Geometry check sheet. Reference: drawing and pictorial views, mm from the part's lowest x, y, z. A direction names the side the tool comes from. Coordinates: 2 decimals unless noted, no trailing zeros. Write each loop counter-clockwise with the first axis right and the second up, starting at its lowest first coordinate (ties: lowest second). Pieces come first, ordered by that corner, then holes. Notation, with made-up numbers: M 29.25,4.25 L 70.25,4.25 A36 ccw 70.25,39.25 Z; hole C 39,-22.75 d7. An arc over 180 degrees is marked long. One line per item, written item: value.
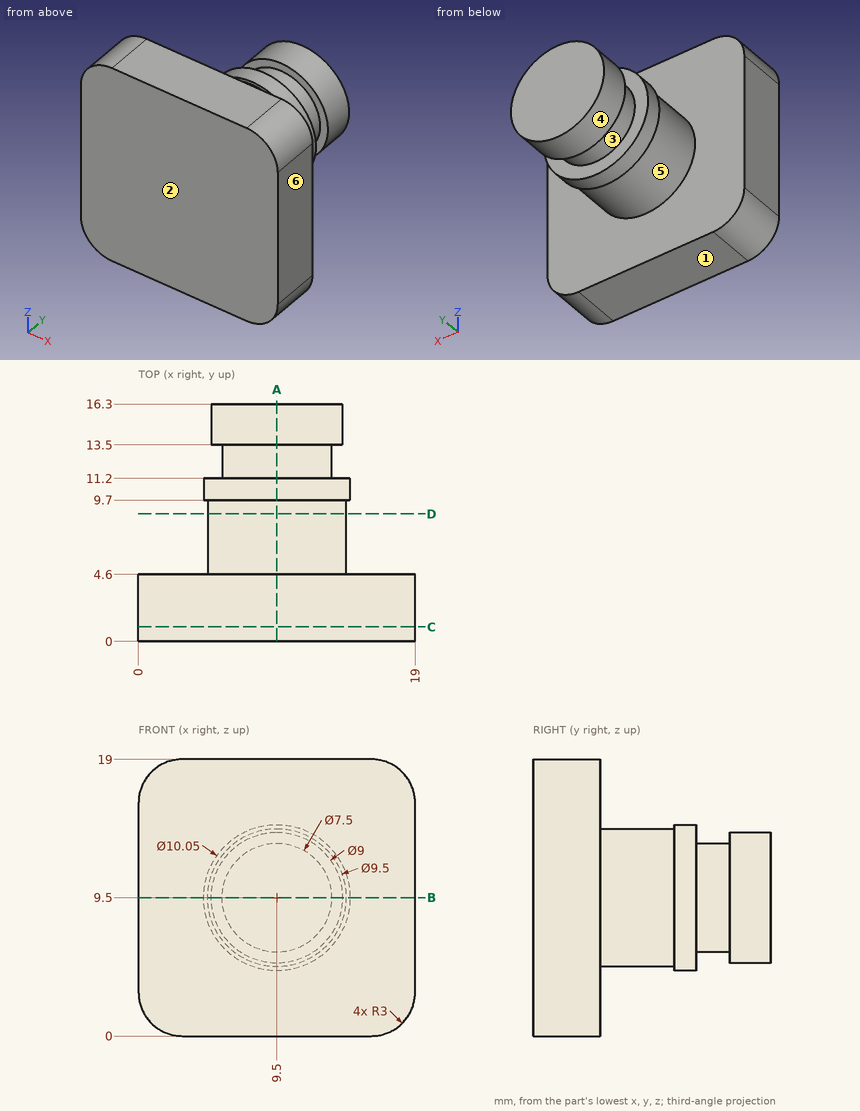
Item 1: Draft check along Y on the marked faces 1, 2 and 3. Enter one of: released by +Y, released by -Y, zero draft, split by the parting line, or undercut.
The answers:
face 1: zero draft
face 2: released by -Y
face 3: undercut
Item 2: Access from +Z, -Z, +X, -X, +Y, -Y to the whole of each face (thin tool, end or side, straight path). Record for the marked faces 4, 5 and 6.
The answers:
face 4: +Y
face 5: none
face 6: +Z, -Z, +X, +Y, -Y
Item 3: Go/stop test with flat-tipped pins: P1, Ø5, axis at x = 11, y = 2.5, coming from the -Z side; P2, Ø4, axis at x = 16.5, y = 12, coming from the -Z side; P3, Ø1, axis at x = 8.5, y = 9.5, coming from the +Z side; P4, Ø5, axis at y = 13, z = 10.5, coming from the +X side (3 decimals). Record where each tip stops, or that it passes through.
The answers:
P1: stops at z = 0
P2: passes through
P3: stops at z = 14.5
P4: stops at x = 14.525
Item 4: Cross-section at C-C, the plane y = 1. Enter the section's corners in (x, z), and give its area (3 significant figures).
The answers:
outline: M 0,3 A3 ccw 3,0 L 16,0 A3 ccw 19,3 L 19,16 A3 ccw 16,19 L 3,19 A3 ccw 0,16 Z
area: 353 mm²
Item 5: Cross-section at B-B, the plane z = 9.5. Enter the section's corners in (x, y) (3 decimals).
The answers:
outline: M 0,0 L 19,0 L 19,4.6 L 14.25,4.6 L 14.25,9.7 L 14.525,9.7 L 14.525,11.2 L 13.25,11.2 L 13.25,13.5 L 14,13.5 L 14,16.3 L 5,16.3 L 5,13.5 L 5.75,13.5 L 5.75,11.2 L 4.475,11.2 L 4.475,9.7 L 4.75,9.7 L 4.75,4.6 L 0,4.6 Z
Item 6: Scan lines: line 1 (Y direction, x = 5.5, z = 16.5); line 2 (X direction, y = 5, z = 11.5); line 3 (Z direction, x = 9.25, y = 10.5). Record each from-to range of solid material in increasing order.
The answers:
line 1: y = 0 to 4.6
line 2: x = 5.19 to 13.81
line 3: z = 4.48 to 14.52
Item 7: Cross-section at D-D, the plane y = 8.75. Enter the section's corners in (x, z), and give its area (3 significant figures).
The answers:
outline: C 9.5,9.5 d9.5
area: 70.9 mm²
Item 8: Cross-section at A-A, the plane x = 9.5. Enter the section's corners in (y, z) (3 decimals), and give its area (3 significant figures).
The answers:
outline: M 0,0 L 4.6,0 L 4.6,4.75 L 9.7,4.75 L 9.7,4.475 L 11.2,4.475 L 11.2,5.75 L 13.5,5.75 L 13.5,5 L 16.3,5 L 16.3,14 L 13.5,14 L 13.5,13.25 L 11.2,13.25 L 11.2,14.525 L 9.7,14.525 L 9.7,14.25 L 4.6,14.25 L 4.6,19 L 0,19 Z
area: 193 mm²
